Read the model definition and answer for the solid it produces. Units are mm, in the model's axes. Face numbers are marked on the shaded views. A direction names the side the tool comes from. Give positions to 0.01 mm unless a question says otherwise; leave off trailing zeros. Order: outer loops, then holes, each group sorted by start corner. A loop starts at its lowest first (then second) coordinate and runs counter-clockwise, first axis right, second up. Notation, with made-up numbers: (-34, -8.75) - (21, -8.75) arc R38 ccw to (21, 29.25) - close; hole circle Ø2 at (83, 58). An arc over 180 degrees is marked (long way). Use a Markdown table: item, result. Add a question column.
1. A cutting plane is placed at C-C on x = 2. Determine the outline of the cut face in (y, z), and give its area (3 significant figures).
2. A cutting plane is placed at B-B on z = 3.85. Determine the outline of the cut face in (x, y), and give its area (4 significant figures).
3. A cutting plane is placed at A-A on y = 1.8. Determine the outline of the cut face in (x, z), and give its area (3 significant figures).
4. A cutting plane is placed at D-D on z = 0.8. Determine the outline of the cut face in (x, y).
5. Flat-ended cylindrical pins translate along their axes: P1, Ø2, axis at y = 2, z = 4.5, coming from the +X side; P2, Ø0.6, axis at y = -0.5, z = 4.5, coming from the +X side; P3, Ø0.6, axis at x = 0, z = 4.5, coming from the +Y side. Find the tip coordinate at first contact, or state that the pin passes through.
6. For a pull along Y with two mould halves and no side action, classify the marked faces 3, 4 and 5 as released by +Y, released by -Y, zero draft, split by the parting line, or undercut.
7. Consider L1, parallel to X at y = 0.1, z = 4.45; L2, parallel to Z at x = 2, y = 0.65. Determine where each line is inside the solid, lowest interval first.
8. Which of the six approach directions +Z, -Z, +X, -X, +Y, -Y give full straight-line access (tool end or side, diameter ignored) to the marked faces 1 and 2?
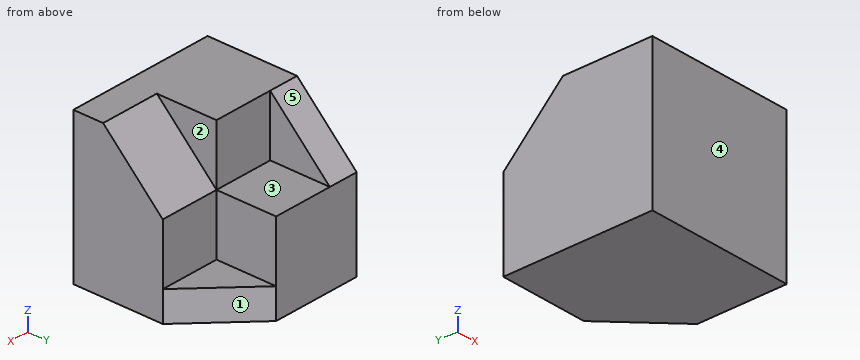
```python
from build123d import *

# Parameters (mm, degrees)
SKETCH1_W           = 5
SKETCH1_H           = 5
BOSS_EXTRUDE1_DEPTH = 5
SKETCH2_W           = 4
SKETCH2_H           = 2
CUT_EXTRUDE1_DEPTH  = 2
SKETCH3_W           = 2
SKETCH3_H           = 2
CUT_EXTRUDE2_DEPTH  = 2
CUT_EXTRUDE3_DEPTH  = 2
CUT_EXTRUDE4_DEPTH  = 2
CUT_EXTRUDE5_DEPTH  = 2


with BuildPart() as part:
    # Sketch1 → Boss-Extrude1 (new body)
    with BuildSketch(Plane.XY):
        Rectangle(SKETCH1_W, SKETCH1_H)
    extrude(amount=BOSS_EXTRUDE1_DEPTH)

    # Sketch2 → Cut-Extrude1 (cut)
    with BuildSketch(Plane(origin=(0, 2.5, 0), x_dir=(1, 0, 0), z_dir=(0, 1, 0))):
        with Locations((0.5, -4)):
            Rectangle(SKETCH2_W, SKETCH2_H)
    extrude(amount=-CUT_EXTRUDE1_DEPTH, mode=Mode.SUBTRACT)

    # Sketch3 → Cut-Extrude2 (cut)
    with BuildSketch(Plane(origin=(0, 2.5, 0), x_dir=(1, 0, 0), z_dir=(0, 1, 0))):
        with Locations((1.5, -2)):
            Rectangle(SKETCH3_W, SKETCH3_H)
    extrude(amount=-CUT_EXTRUDE2_DEPTH, mode=Mode.SUBTRACT)

    # Sketch4 → Cut-Extrude3 (cut, through all)
    with BuildSketch(Plane.XY.offset(1)):
        Polygon((0.5, 2.5), (2.5, 0.5), (2.5, 2.5), align=None)
    extrude(amount=-CUT_EXTRUDE3_DEPTH, mode=Mode.SUBTRACT)

    # Sketch5 → Cut-Extrude4 (cut)
    with BuildSketch(Plane(origin=(2.5, 0, 0), x_dir=(0, 0, -1), z_dir=(1, 0, 0))):
        Polygon((-5, 0.5), (-3, 0.5), (-5, -1.5), align=None)
    extrude(amount=-CUT_EXTRUDE4_DEPTH, mode=Mode.SUBTRACT)

    # Sketch6 → Cut-Extrude5 (cut, through all)
    with BuildSketch(Plane(origin=(-1.5, 0, 0), x_dir=(0, 0, -1), z_dir=(1, 0, 0))):
        Polygon((-3, 2.5), (-5, 0.5), (-5, 2.5), align=None)
    extrude(amount=-CUT_EXTRUDE5_DEPTH, mode=Mode.SUBTRACT)


solid = part.part
```
Output values:
| question | item | result |
|---|---|---|
| 1 | outline | (-2.5, 0) - (1, 0) - (1, 1) - (0.5, 1) - (0.5, 3) - (-1.5, 5) - (-2.5, 5) - close |
| 1 | area | 13.5 mm² |
| 2 | outline | (-2.5, -2.5) - (2.5, -2.5) - (2.5, -0.35) - (0.5, -0.35) - (0.5, 0.5) - (-1.5, 0.5) - (-1.5, 1.65) - (-2.5, 1.65) - close |
| 2 | area | 14.45 mm² |
| 3 | outline | (-2.5, 0) - (1.2, 0) - (1.2, 1) - (0.5, 1) - (0.5, 3) - (-1.5, 3) - (-1.5, 3.7) - (-2.5, 3.7) - close |
| 3 | area | 10.4 mm² |
| 4 | outline | (-2.5, -2.5) - (2.5, -2.5) - (2.5, 0.5) - (0.5, 2.5) - (-2.5, 2.5) - close |
| 5 | P1 | x = -1.5 |
| 5 | P2 | x = 0.5 |
| 5 | P3 | y = 0.5 |
| 6 | face 3 | zero draft |
| 6 | face 4 | released by -Y |
| 6 | face 5 | released by +Y |
| 7 | L1 | -2.5 to 0.5 |
| 7 | L2 | 0 to 1 |
| 8 | face 1 | +Z, -Z, +X, +Y |
| 8 | face 2 | +Z, +X, +Y |
